The model under review builds one solid part; all positions refer to its coordinate system, in mm. Face numbers are marked on the shaded views. Coordinates: 2 decimals unless noted, no trailing zeros. Write each loop counter-clockwise with the first axis right and the second up, starting at its lowest first coordinate (ties: lowest second). Pieces come first, ordered by that corner, then holes. Notation, with made-up numbers: (74.5, 66.25) - (78.5, 66.25) arc R36 ccw to (78.5, 103.25) - close; hole circle Ø6 at (60, 6.25). An arc over 180 degrees is marked (long way). Put each result on its own line as item: value. Start each with the question number.
Item 1: To check wall thickness, follow L1, parallel to Z at x = 0, y = 17; L2, parallel to Y at x = 11.5, z = -3.5; L3, parallel to Z at x = 36, y = -31.5. State the ranges of each line that lie inside material, in increasing order. Write a range as [from, to].
Item 2: Consider section A-A on y = -25.5. Give the boundary of the cut face in (x, z), then the cut area to 3 significant figures.
Item 3: For pin 1 (1.5 mm diameter, centred on y = 17, z = -9.5, fed in from -X); pin 2 (1.5 mm diameter, centred on x = 16.5, y = -29, fed in from +Z); pin 3 (1.5 mm diameter, centred on y = 17, z = 8, fed in from -X), all flat-tipped, find the tip position at first contact; note any pin that passes through.
Item 4: Mouldability with a two-part tool opening along X and no side actions: class the marked faces 1, 2 and 3 as pulls with the +X half, pulls with the -X half, needs draft (parallel to the pull), parting line crosses it, or undercut.
```python
from build123d import *

# Parameters (mm, degrees)
SHELL2_T  = -1
FILLET1_R = 2
FILLET2_R = 1


with BuildPart() as part:
    # Sketch1 → Revolve1 (revolve)
    with BuildSketch(Plane.XY, mode=Mode.PRIVATE) as revolve1_sk:
        Polygon((0, -38.642009768), (40, -38.642009768), (40, 48.926842765), (42.431147467, 51.357990232), (0, 51.357990232), align=None)
    revolve(revolve1_sk.sketch.rotate(Axis((0, 51.357990232, 0), (0, -1, 0)), 180), axis=Axis((0, 51.357990232, 0), (0, -1, 0)))

    # Shell2
    shell2_openings = [part.faces().sort_by_distance(p)[0] for p in [
        (0, 51.357990232, 0),
    ]]
    offset(amount=SHELL2_T, openings=shell2_openings, kind=Kind.INTERSECTION)

    # Fillet1
    fillet1_edges = [part.edges().sort_by_distance(p)[0] for p in [
        (40, -38.642009768, 0),
    ]]
    fillet(fillet1_edges, radius=FILLET1_R)

    # Fillet2
    fillet2_edges = [part.edges().sort_by_distance(p)[0] for p in [
        (40, 48.926842765, 0),
    ]]
    fillet(fillet2_edges, radius=FILLET2_R)


solid = part.part
```
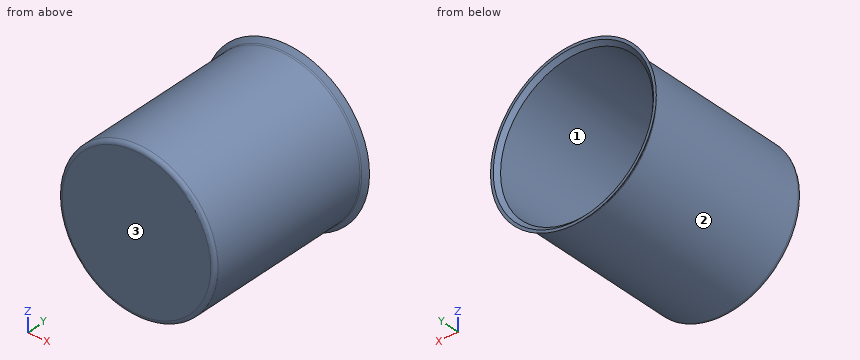
Report:
1. L1: [-40, -39], [39, 40]
1. L2: [-38.64, -37.64]
1. L3: [-17.44, -15], [15, 17.44]
2. outline: circle Ø80 at (0, 0); hole circle Ø78 at (0, 0)
2. area: 248 mm²
3. pin 1: x = -39.03
3. pin 2: z = 36.77
3. pin 3: x = -39.34
4. face 1: undercut
4. face 2: parting line crosses it
4. face 3: needs draft
